from build123d import *

# Parameters (mm, degrees)
BOSS_EXTRUDE1_DEPTH = 2.5
SKETCH1_3_W         = 3.753393981
SKETCH1_3_H         = 3
SKETCH1_3_W_2       = 4.246606019
SKETCH1_3_H_2       = 2.7
SKETCH1_3_W_3       = 8
BOSS_EXTRUDE2_DEPTH = 3.15


with BuildPart() as part:
    # Sketch1 → Boss-Extrude1 (new body)
    with BuildSketch(Plane.XY):
        Polygon((12.375, 4), (-12.375, 4), (-12.375, 1), (-12.375, -1.3), (-12.375, -4), (12.375, -4), (12.375, -1.3), (12.375, 1), align=None)
    extrude(amount=BOSS_EXTRUDE1_DEPTH)

    # Sketch1<3> → Boss-Extrude2 (add)
    with BuildSketch(Plane.XY):
        with Locations((-18.498303009, 2.5)):
            Rectangle(SKETCH1_3_W, SKETCH1_3_H)
        with Locations((-14.49830301, 2.5)):
            Rectangle(SKETCH1_3_W_2, SKETCH1_3_H)
        with Locations((-14.49830301, -2.65)):
            Rectangle(SKETCH1_3_W_2, SKETCH1_3_H_2)
        with Locations((-18.498303009, -2.65)):
            Rectangle(SKETCH1_3_W, SKETCH1_3_H_2)
        with Locations((16.375, -2.65)):
            Rectangle(SKETCH1_3_W_3, SKETCH1_3_H_2)
        with Locations((16.375, 2.5)):
            Rectangle(SKETCH1_3_W_3, SKETCH1_3_H)
    extrude(amount=BOSS_EXTRUDE2_DEPTH)


solid = part.part
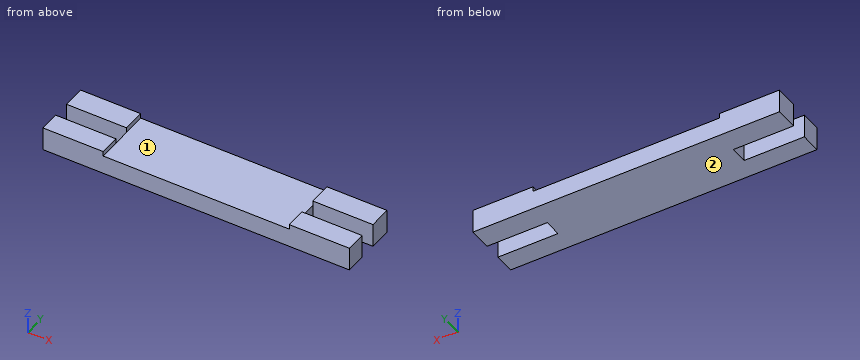
Work out the finished part from the listing and answer in its coordinate system (mm). Face numbers are marked on the shaded views. Round coordinates to 2 decimals unless told otherwise and drop trailing zeros. Write each loop counter-clockwise with the first axis right and the second up, starting at its lowest first coordinate (ties: lowest second). Pieces come first, ordered by that corner, then holes.
1) A cutting plane is placed at C-C (z = 1.15). Give the vertices of the cut face in (x, y) (3 decimals).
2) Straight lines are drawn through the part: line 1 (Y direction, x = 13.5, z = 0.9); line 2 (X direction, y = 2, z = 2.75) (3 decimals); line 3 (Z direction, x = -6.5, y = -1.5). For each, find the intervals that lie inside material, in ascending order.
3) Given pin 1 Ø1 at (x, y) = (-11.5, 0.5) entering from +Z; pin 2 Ø1.8 at (y, z) = (0, 1.5) entering from -X (3 decimals), each flat-ended and moving along its own axis, determine where each tip first touches the part or whether it passes through.
4) The mould has two halves that part along X. Classify the marked faces 1 and 2: pulls with the +X half, pulls with the -X half, needs draft (parallel to the pull), parting line crosses it, or undercut.
5) A cutting plane is placed at A-A (x = 18). Give the vertices of the cut face in (y, z).
6) A cutting plane is placed at D-D (x = 10.5). Give the vertices of the cut face in (y, z).
7) A cutting plane is placed at B-B (y = -2.5). Give the vertices of the cut face in (x, z) (3 decimals), plus the area to 3 significant figures.
Completed:
1. outline: (-20.375, -4) - (20.375, -4) - (20.375, -1.3) - (12.375, -1.3) - (12.375, 1) - (20.375, 1) - (20.375, 4) - (-20.375, 4) - (-20.375, 1) - (-12.375, 1) - (-12.375, -1.3) - (-20.375, -1.3) - close
2. line 1: y = -4 to -1.3, 1 to 4
2. line 2: x = -20.375 to -12.375, 12.375 to 20.375
2. line 3: z = 0 to 2.5
3. pin 1: stops at z = 2.5
3. pin 2: stops at x = -12.375
4. face 1: undercut
4. face 2: needs draft
5. outline: (-4, 0) - (-1.3, 0) - (-1.3, 3.15) - (-4, 3.15) - close; (1, 0) - (4, 0) - (4, 3.15) - (1, 3.15) - close
6. outline: (-4, 0) - (4, 0) - (4, 2.5) - (-4, 2.5) - close
7. outline: (-20.375, 0) - (20.375, 0) - (20.375, 3.15) - (12.375, 3.15) - (12.375, 2.5) - (-12.375, 2.5) - (-12.375, 3.15) - (-20.375, 3.15) - close
7. area: 112 mm2
